Could you check a few things on this model? Use its own coordinates, in mm. A direction names the side the tool comes from. Give positions to 0.01 mm unless a question says otherwise; leave off trailing zeros. Order: outer loops, then holes, each group sorted by start corner. A loop starts at its lowest first (then second) coordinate and runs counter-clockwise, first axis right, second up. Notation, with made-up numbers: (54, 44.5) -> (82, 44.5) arc R19 cw to (82, 77.5) -> close; hole circle Ø8 at (-21.75, -18.5). An arc over 180 degrees is marked (long way). Answer as CSV lines item,"result". Start each with the question number.
(1) I want a section at B-B (z = 0). Please give me the cut outline in (x, y), plus the area to 3 significant figures.
(2) I want a section at A-A (y = 0). Please give me the cut outline in (x, z).
(3) I want a section at D-D (z = 9.25). Please give me the cut outline in (x, y), plus the area to 3 significant figures.
(4) On a 3-axis mill with a long thin cutter (end or side, diameter ignored), from which of +Z, -Z, +X, -X, +Y, -Y can I reach the whole of each face in a straight line? I mean faces 4 (the face through (2, 9.398, 0)), 5 (the face through (24.306, -1.363, 6.137)). Say none if no direction works.
(5) I want a section at C-C (x = 10.5). Please give me the cut outline in (y, z).
(6) Will these pins go through, and if not, where does the flat tip stop? pin 1 Ø6 at (x, z) = (13, -3.5) entering from +Y; pin 2 Ø1.5 at (x, z) = (27.5, -5.5) entering from -Y; pin 3 Ø4 at (x, y) = (5.5, 2.5) entering from -Z; pin 4 Ø5 at (y, z) = (-6.5, 2) entering from -X.
(7) We'd pull the mould along Z, two halves only. Please class faces 1 (the face through (2.35, -0.15, 11.43)), 2 (the face through (21.142, -3.186, -0.708)), 3 (the face through (42.862, -1.3, 4.1)): released by +Z, released by -Z, zero draft, split by the parting line, or undercut.
(8) I need wall thicknesses on L1, parallel to Y at x = 14, z = 0; L2, parallel to X at y = -4.75, z = 6; L3, parallel to Z at x = 4.5, y = 6.5. Which ranges of each line are inside material? Lowest first, please.
```python
from build123d import *

# Parameters (mm, degrees)
FILLET1_R             = 1.5
HOLE_WIZARD_5_16_18_D = 6.5278
CUT_EXTRUDE1_DEPTH    = 43.8625
CHAMFER1_SIZE         = 0.762


with BuildPart() as part:
    # Sketch1 → Revolve1 (revolve)
    with BuildSketch(Plane.XY):
        Polygon((0, 0), (42.8625, 0), (42.8625, 6.2865), (4.7625, 6.2865), (4.7625, 11.43), (0, 11.43), align=None)
    revolve(axis=Axis((0, 0, 0), (-1, 0, 0)))

    # Fillet1
    fillet1_edges = [part.edges().sort_by_distance(p)[0] for p in [
        (4.7625, -6.2865, 0),
    ]]
    fillet(fillet1_edges, radius=FILLET1_R)

    # 5/16-18 (through all)
    with Locations(Plane(origin=(42.8625, 0, 0), x_dir=(0, 0, -1), z_dir=(1, 0, 0))):
        with Locations((0, 0)):
            Hole(HOLE_WIZARD_5_16_18_D / 2)

    # Sketch4 → Cut-Extrude1 (cut, through all)
    with BuildSketch(Plane.ZY):
        with BuildLine():
            Line((-6.505574225, 9.398), (6.505574225, 9.398))
            ThreePointArc((6.505574225, 9.398), (0, 11.43), (-6.505574225, 9.398))
        make_face()
        with BuildLine():
            Line((6.505574225, -9.398), (-6.505574225, -9.398))
            ThreePointArc((-6.505574225, -9.398), (0, -11.43), (6.505574225, -9.398))
        make_face()
    extrude(amount=-CUT_EXTRUDE1_DEPTH, mode=Mode.SUBTRACT)

    # Chamfer1
    chamfer1_edges = [part.edges().sort_by_distance(p)[0] for p in [
        (42.8625, 0, -3.2639),
        (0, 0, -3.2639),
    ]]
    chamfer(chamfer1_edges, length=CHAMFER1_SIZE)


solid = part.part
```
Final values:
1,outline,"(0, -9.4) -> (4.76, -9.4) -> (4.76, -7.79) arc R1.5 cw to (6.26, -6.29) -> (42.86, -6.29) -> (42.86, -4.03) -> (42.1, -3.26) -> (0.76, -3.26) -> (0, -4.03) -> close; (0, 4.03) -> (0.76, 3.26) -> (42.1, 3.26) -> (42.86, 4.03) -> (42.86, 6.29) -> (6.26, 6.29) arc R1.5 cw to (4.76, 7.79) -> (4.76, 9.4) -> (0, 9.4) -> close"
1,area,"289 mm²"
2,outline,"(0, -11.43) -> (4.76, -11.43) -> (4.76, -7.79) arc R1.5 cw to (6.26, -6.29) -> (42.86, -6.29) -> (42.86, -4.03) -> (42.1, -3.26) -> (0.76, -3.26) -> (0, -4.03) -> close; (0, 4.03) -> (0.76, 3.26) -> (42.1, 3.26) -> (42.86, 4.03) -> (42.86, 6.29) -> (6.26, 6.29) arc R1.5 cw to (4.76, 7.79) -> (4.76, 11.43) -> (0, 11.43) -> close"
3,outline,"(0, -6.71) -> (4.76, -6.71) -> (4.76, 6.71) -> (0, 6.71) -> close"
3,area,"64.0 mm²"
4,face 4,"+Z, -Z, +X, -X, +Y"
4,face 5,"+X"
5,outline,"circle Ø12.57 at (0, 0); hole circle Ø6.53 at (0, 0)"
6,pin 1,"y = 6.27"
6,pin 2,"y = -4.12"
6,pin 3,"z = -11.41"
6,pin 4,"x = 0"
7,face 1,"released by +Z"
7,face 2,"undercut"
7,face 3,"zero draft"
8,L1,"-6.29 to -3.26, 3.26 to 6.29"
8,L2,"0 to 4.77"
8,L3,"-9.4 to 9.4"
